Autodesk Fusion 360 part; units mm, degrees
sketch "Sketch1" plane through (0, 0, 0) normal (0, 1, 0) x (1, 0, 0)
  circle A0 centre (0, 0) radius 5
  circle A1 centre (0, 0) radius 1.6
  line L0 (-5, 0) -> (5, 0)
  line L1 (5, 0) -> (5, -100.7)
  line L2 (5, -100.7) -> (-5, -100.7)
  line L3 (-5, -100.7) -> (-5, 0)
  circle A2 centre (0, -100.7) radius 5
  circle A3 centre (0, -100.7) radius 1.6
  dimension "d1" = 10
  dimension "d2" = 3.2
  dimension "d3" = 100.7
  dimension "d4" = 3.2
extrude "Extrude1" add sketch "Sketch1" along normal blind 5.9 contours L2 A2 A3 | L2 A2 A3
extrude "Extrude2" add sketch "Sketch1" against normal blind 5 contours A0 A1 L0 | A0 L1 L3 A2 | A0 A1 L0 | L2 A2 A3 | L2 A2 A3
equation "d3 = 106 mm - 20.3 mm + 15 mm"
Geometry: final body of the model. Coordinates: model frame, mm. A direction names the side the tool comes from. Give positions to 0.01 mm unless a question says otherwise; leave off trailing zeros. Order: outer loops, then holes, each group sorted by start corner. A loop starts at its lowest first (then second) coordinate and runs counter-clockwise, first axis right, second up. Notation, with made-up numbers: (37.5, -22) -> (92.5, -22) arc R23 cw to (92.5, -4) -> close; hole circle Ø9 at (41.25, 31). An arc over 180 degrees is marked (long way). Write each question's results on one line, items separated by ' | '. Start each with the question number.
1) Draft query along X for faces 3 (the flat face through (5, -2, 50)), 4 (the cylindrical face through (0.86, 0.37, 102.05)), 5 (the flat face through (2, 5.9, 101)). Return one class per face: pulls with the +X half, pulls with the -X half, needs draft (parallel to the pull), parting line crosses it, or undercut.
2) Section C-C (z = 31). Return loops of the section in (x, y), then the cut area to 3 significant figures.
3) First-contact query: pin 1 (5 mm diameter, centred on x = 0, z = 0, fed in from +Y); pin 2 (1 mm diameter, centred on x = -1.5, y = 4.5, fed in from -Z); pin 3 (2 mm diameter, centred on x = -1.5, y = 0.5, fed in from +Z). Flat tips, straight axial feed; report the tip coordinate or a pass-through.
4) Line query: line 1 (Z direction, x = 0, y = -3.75); line 2 (X direction, y = 1.5, z = 100.7); line 3 (Y direction, x = 3, z = 19.5). Output: solid intervals per line, ascending. Write a range as from..to.
5) Set-up query: faces 1 (the flat face through (0, -5, 50)), 2 (the cylindrical face through (-0.651, 1.585, 105.657)). Return all of +Z, -Z, +X, -X, +Y, -Y with unobstructed straight access to the full face (end or side cutting, diameter ignored); none if empty.
6) Section A-A (x = 0). Return loops of the section in (y, z), then the cut area to 3 significant figures.
7) Section B-B (y = 5). Return loops of the section in (x, z).
Calculated:
1) face 3: pulls with the +X half | face 4: undercut | face 5: needs draft
2) outline: (-5, -5) -> (5, -5) -> (5, 0) -> (-5, 0) -> close | area: 50.0 mm2
3) pin 1: y = 0 | pin 2: z = 95.8 | pin 3: z = 105.67
4) line 1: -5..-1.6, 1.6..99.1, 102.3..105.7 | line 2: -5..-1.6, 1.6..5 | line 3: -5..0
5) face 1: +Z, -Z, +X, -X, -Y | face 2: +Y
6) outline: (-5, -5) -> (0, -5) -> (0, -1.6) -> (-5, -1.6) -> close; (-5, 1.6) -> (0, 1.6) -> (0, 95.7) -> (5.9, 95.7) -> (5.9, 99.1) -> (-5, 99.1) -> close; (-5, 102.3) -> (5.9, 102.3) -> (5.9, 105.7) -> (-5, 105.7) -> close | area: 562 mm2
7) outline: circle Ø10 at (0, 100.7); hole circle Ø3.2 at (0, 100.7)
